CAD build for the part. Positions are in the model's coordinates, mm. Round coordinates to 2 decimals unless told otherwise and drop trailing zeros. Answer as CSV lines item,"result". Start each with the question number.
```python
from build123d import *

# Parameters (mm, degrees)
SKETCH1_R           = 12.7
BOSS_EXTRUDE1_DEPTH = 1.27
SKETCH2_R           = 9.525
BOSS_EXTRUDE2_DEPTH = 2.54
SKETCH3_R           = 12.7
BOSS_EXTRUDE3_DEPTH = 1.27
SHELL1_OUTLINE_R    = 8.255
SHELL1_DEPTH        = 5.08
FILLET1_R           = 2.54
FILLET2_R           = 2.54


# Read off the part's stored shape, not the designer's step: Shell1
# Some blends are built 0.0001 mm under size
with BuildPart() as part:
    # Sketch1 → Boss-Extrude1 (new body)
    with BuildSketch(Plane(origin=(0, 0, 0), x_dir=(1, 0, 0), z_dir=(0, 1, 0))):
        with Locations(Location((0, 0, 0), (0, 0, 270))):
            Circle(SKETCH1_R)
    extrude(amount=BOSS_EXTRUDE1_DEPTH)

    # Sketch2 → Boss-Extrude2 (add)
    with BuildSketch(Plane(origin=(0, 1.27, 0), x_dir=(1, 0, 0), z_dir=(0, 1, 0))):
        with Locations(Location((0, 0, 0), (0, 0, 270))):
            Circle(SKETCH2_R)
    extrude(amount=BOSS_EXTRUDE2_DEPTH)

    # Sketch3 → Boss-Extrude3 (add)
    with BuildSketch(Plane(origin=(0, 3.81, 0), x_dir=(1, 0, 0), z_dir=(0, 1, 0))):
        with Locations(Location((0, 0, 0), (0, 0, 270))):
            Circle(SKETCH3_R)
    extrude(amount=BOSS_EXTRUDE3_DEPTH)

    # Shell1 outline → Shell1 (cut)
    with BuildSketch(Plane(origin=(0, 0, 0), x_dir=(1, 0, 0), z_dir=(0, 1, 0))):
        Circle(SHELL1_OUTLINE_R)
    extrude(amount=SHELL1_DEPTH, mode=Mode.SUBTRACT)

    # Fillet1
    # the kernel refuses this fillet: 2.54 mm, written as the material it takes off along each edge
    with BuildSketch(Plane(origin=(0, 1.27, 0), x_dir=(0, 0, 1), z_dir=(-1, 0, 0))) as fillet1_piece_1:
        with BuildLine():
            CenterArc((10.500295474, -2.54), FILLET1_R, 30, 60)
            Line((12.7, -1.27), (12.743994091, -1.2446))
            ThreePointArc((12.743994091, -1.2446), (12.7508, -0.635), (12.7508, 0))
            Line((12.7508, 0), (12.7, 0.0508))
            Line((12.7, 0.0508), (10.500295474, 0.0508))
            Line((10.500295474, 0.0508), (10.500295474, 0))
        make_face()
    revolve(axis=Axis((0, 1.27, 0), (0, 1, 0)), mode=Mode.SUBTRACT)
    with BuildSketch(Plane(origin=(0, 3.81, 0), x_dir=(0, 0, 1), z_dir=(-1, 0, 0))) as fillet1_piece_2:
        with BuildLine():
            CenterArc((10.500295474, 2.54), FILLET1_R, 270, 60)
            Line((10.500295474, 0), (10.500295474, -0.0508))
            Line((10.500295474, -0.0508), (12.7, -0.0508))
            Line((12.7, -0.0508), (12.7508, 0))
            ThreePointArc((12.7508, 0), (12.7508, 0.635), (12.743994091, 1.2446))
            Line((12.743994091, 1.2446), (12.7, 1.27))
        make_face()
    revolve(axis=Axis((0, 3.81, 0), (0, 1, 0)), mode=Mode.SUBTRACT)

    # Fillet2
    fillet2_edges = [part.edges().sort_by_distance(p)[0] for p in [
        (-8.255, 5.08, 0),
        (-8.255, 0, 0),
    ]]
    fillet(fillet2_edges, radius=FILLET2_R - 0.0001)  # a hair under: the kernel refuses the full size


solid = part.part
```
Q1. Drop flat-ended pins along their axis: P1, Ø10.5, axis at x = 3, z = 4, coming from the +Y side; P2, Ø1, axis at x = 8, y = 3, coming from the +Z side; P3, Ø2, axis at y = 2.5, z = 7, coming from the -X side. Give the stop position or say it passes through.
Q2. Probe line 1 along X through (y, z) = (2.5, 0) (3 decimals); line 2 along Y through (x, z) = (-6.25, -9.25); line 3 along X through (y, z) = (4.25, 0.5). List the from-to ranges inside material, lowest first. Write a range as from..to.
Q3. Mould opens along Y. For faces 1 (the cylindrical face through (-5.796, 2.522, -7.559)), 2 (the flat face through (-9.35, 0, -5.7)), 3 (the flat face through (-9.35, 5.08, -5.7)) say: +Y half, -Y half, draft (parallel to the pull), parting line (faces both ways), or undercut.
Answer:
1,P1,"stops at y = 5.02"
1,P2,"stops at z = 5.87"
1,P3,"stops at x = -7.4"
2,line 1,"x = -9.525..-8.255, 8.255..9.525"
2,line 2,"y = 0..1.18, 3.9..5.08"
2,line 3,"x = -11.92..-8.9, 8.9..11.92"
3,face 1,"undercut"
3,face 2,"-Y half"
3,face 3,"+Y half"
